```python
from build123d import *

# Parameters (mm, degrees)
SKETCH1_R           = 3.25
BOSS_EXTRUDE2_DEPTH = 4
SKETCH2_R           = 6.5
SKETCH2_R_2         = 3.25
BOSS_EXTRUDE3_DEPTH = 4
SKETCH3_R           = 3.25
CUT_EXTRUDE1_DEPTH  = 10


with BuildPart() as part:
    # Sketch1 → Boss-Extrude2 (new body)
    with BuildSketch(Plane.XY):
        with BuildLine():
            Line((4, -4.472135955), (4, 4.472135955))
            ThreePointArc((4, 4.472135955), (-6, 0), (4, -4.472135955))
        make_face()
        Circle(SKETCH1_R, mode=Mode.SUBTRACT)
        with BuildLine():
            ThreePointArc((6, 0), (5.477225575, 2.449489743), (4, 4.472135955))
            Line((4, 4.472135955), (4, -4.472135955))
            ThreePointArc((4, -4.472135955), (5.477225575, -2.449489743), (6, 0))
        make_face()
        with BuildLine():
            Line((90, 4.472135955), (4, 4.472135955))
            ThreePointArc((4, 4.472135955), (5.477225575, 2.449489743), (6, 0))
            ThreePointArc((6, 0), (5.477225575, -2.449489743), (4, -4.472135955))
            Line((4, -4.472135955), (90, -4.472135955))
            Line((90, -4.472135955), (90, 4.472135955))
        make_face()
    extrude(amount=BOSS_EXTRUDE2_DEPTH)

    # Sketch2 → Boss-Extrude3 (add)
    with BuildSketch(Plane.XY.offset(4)):
        with Locations((90, 0)):
            Circle(SKETCH2_R)
        with Locations((90, 0)):
            Circle(SKETCH2_R_2, mode=Mode.SUBTRACT)
    extrude(amount=-BOSS_EXTRUDE3_DEPTH)

    # Sketch3 → Cut-Extrude1 (cut)
    with BuildSketch(Plane.XY.offset(4)):
        with Locations((90, 0)):
            Circle(SKETCH3_R)
    extrude(amount=-CUT_EXTRUDE1_DEPTH, mode=Mode.SUBTRACT)


solid = part.part
```
Input: part model. Units: mm. Frame: model coordinates. A direction names the side the tool comes from. Give positions to 0.01 mm unless a question says otherwise; leave off trailing zeros. Loops run counter-clockwise (first coordinate to the right, second up) from the corner with the lowest first, then second, coordinate; pieces in that order, holes last. Notation, with made-up numbers: (25, 57.25) -> (82, 57.25) arc R11 cw to (82, 77.25) -> close; hole circle Ø2 at (11.25, 48). An arc over 180 degrees is marked (long way). Use a Markdown table: item, result.
Q1. Section query C-C, the plane z = 2.5. Return the cut outline in (x, y), plus the area to 3 significant figures.
Entries:
| item | result |
|---|---|
| outline | (4, -4.47) -> (85.28, -4.47) arc R6.5 ccw (long way) to (85.28, 4.47) -> (4, 4.47) arc R6 ccw (long way) to start; hole circle Ø6.5 at (0, 0); hole circle Ø6.5 at (90, 0) |
| area | 883 mm² |
Q2. Pull-direction query (X, two-part tool) for faces 1 (the flat face through (45, 0, 4)), 2 (the cylindrical face through (87.26, 1.75, 2.03)); classes: pulls with the +X half, pulls with the -X half, needs draft (parallel to the pull), parting line crosses it, or undercut.
Entries:
| item | result |
|---|---|
| face 1 | needs draft |
| face 2 | undercut |
Q3. Section query A-A, the plane x = 0. Return the cut outline in (y, z).
Entries:
| item | result |
|---|---|
| outline | (-6, 0) -> (-3.25, 0) -> (-3.25, 4) -> (-6, 4) -> close; (3.25, 0) -> (6, 0) -> (6, 4) -> (3.25, 4) -> close |
Q4. First-contact query: P1, Ø1, axis at x = 62.5, z = 1, coming from the +Y side; P2, Ø3, axis at x = 19, y = -0.5, coming from the -Z side; P3, Ø1.5, axis at x = 38, z = 2, coming from the -Y side; P4, Ø2, axis at y = 1.5, z = 2, coming from the -X side. Flat tips, straight axial feed; report the tip coordinate or a pass-through.
Entries:
| item | result |
|---|---|
| P1 | stops at y = 4.47 |
| P2 | stops at z = 0 |
| P3 | stops at y = -4.47 |
| P4 | stops at x = -5.98 |
Q5. Ray query, probe 1 along X at (y, z) = (2, 2.4); probe 2 along Y at (x, z) = (0, 2.85); probe 3 along Y at (x, z) = (47.5, 0.3). Return the intervals inside material, ascending. Write a range as from..to.
Entries:
| item | result |
|---|---|
| probe 1 | x = -5.66..-2.56, 2.56..87.44, 92.56..96.18 |
| probe 2 | y = -6..-3.25, 3.25..6 |
| probe 3 | y = -4.47..4.47 |
Q6. Section query B-B, the plane y = 0. Return the cut outline in (x, z).
Entries:
| item | result |
|---|---|
| outline | (-6, 0) -> (-3.25, 0) -> (-3.25, 4) -> (-6, 4) -> close; (3.25, 0) -> (86.75, 0) -> (86.75, 4) -> (3.25, 4) -> close; (93.25, 0) -> (96.5, 0) -> (96.5, 4) -> (93.25, 4) -> close |
Q7. Access query for faces 3 (the flat face through (44, -4.472, 2)), 4 (the flat face through (45, 4.472, 2)), 5 (the cylindrical face through (-2.579, -1.978, 1.972)). Directions: +Z, -Z, +X, -X, +Y, -Y. A direction counts if a zero-diameter tool reaches every point of the face in a straight line with its end or side. Return the directions, or none.
Entries:
| item | result |
|---|---|
| face 3 | +Z, -Z, -Y |
| face 4 | +Z, -Z, +Y |
| face 5 | +Z, -Z |
Q8. Section query D-D, the plane x = 90. Return the cut outline in (y, z), plus the area to 3 significant figures.
Entries:
| item | result |
|---|---|
| outline | (-6.5, 0) -> (-3.25, 0) -> (-3.25, 4) -> (-6.5, 4) -> close; (3.25, 0) -> (6.5, 0) -> (6.5, 4) -> (3.25, 4) -> close |
| area | 26.0 mm² |
